Source: three-view drawing plus pictorial views. Frame: mm from the lowest corner of the part. A direction names the side the tool comes from. Give positions to 0.01 mm unless a question says otherwise; leave off trailing zeros. Loops run counter-clockwise (first coordinate to the right, second up) from the corner with the lowest first, then second, coordinate; pieces in that order, holes last. Notation, with made-up numbers: (10, 59) - (33, 59) arc R23 ccw to (33, 95) - close; hole circle Ø5 at (-14, 31.5). An arc over 180 degrees is marked (long way). Answer as a JSON object with one key per item and string values. Group by question number.
(1) Section query A-A (y = 12). Return loops of the section in (x, z), plus the area to 3 significant figures.
(2) Pin query (flat end, axial travel): P1, Ø1.5, axis at y = 7, z = 17, coming from the -X side; P2, Ø4.5, axis at x = 49.5, y = 17, coming from the -Z side; P3, Ø12, axis at x = 30, z = 20, coming from the +Y side. Return the tip coordinate at first contact, or that it passes through.
(3) Access query for the marked faces 1 and 2. Directions: +Z, -Z, +X, -X, +Y, -Y. A direction counts if a zero-diameter tool reaches every point of the face in a straight line with its end or side. Return the directions, or none.
(4) Section query B-B (z = 20). Return loops of the section in (x, y).
(5) Material intervals for L1, parallel to Y at x = 52.5, z = 44.75; L2, parallel to X at y = 19, z = 20; L3, parallel to Z at x = 49, y = 18.5, sorted ascending.
(6) Mould query, pull axis X, two halves, no side actions, for the marked faces 3, 4, 5 and 6. Classes: +X half, -X half, draft (parallel to the pull), parting line (faces both ways), or undercut.
(7) Section query C-C (x = 30). Return loops of the section in (y, z).
(8) Section query D-D (y = 2.75). Return loops of the section in (x, z).
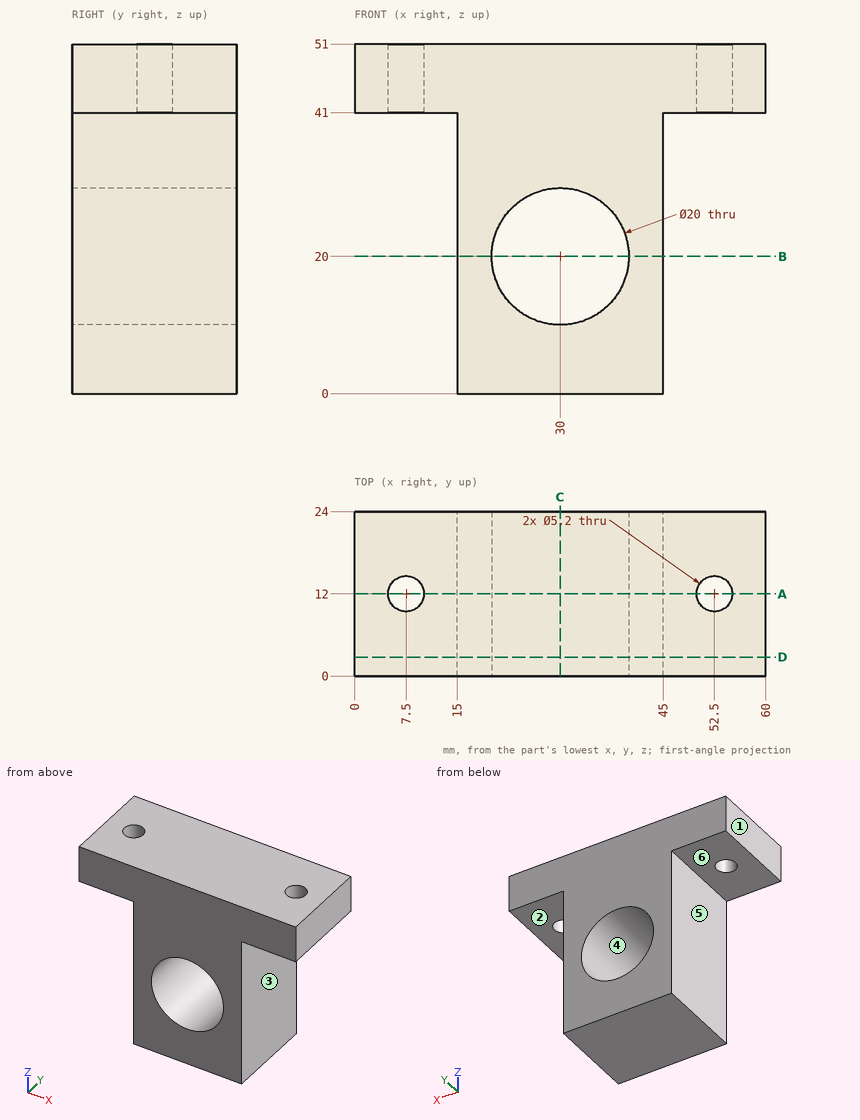
Recorded:
{
 "1": {"outline": "(0, 41) - (4.9, 41) - (4.9, 51) - (0, 51) - close; (10.1, 41) - (15, 41) - (15, 0) - (45, 0) - (45, 41) - (49.9, 41) - (49.9, 51) - (10.1, 51) - close; (55.1, 41) - (60, 41) - (60, 51) - (55.1, 51) - close; hole circle Ø20 at (30, 20)", "area": "1,410 mm^2"},
 "2": {"P1": "stops at x = 15", "P2": "stops at z = 41", "P3": "passes through"},
 "3": {"face 1": "+Z, -Z, -X, +Y, -Y", "face 2": "-Z, +X, +Y, -Y"},
 "4": {"outline": "(15, 0) - (20, 0) - (20, 24) - (15, 24) - close; (40, 0) - (45, 0) - (45, 24) - (40, 24) - close"},
 "5": {"L1": "y = 0 to 9.4, 14.6 to 24", "L2": "x = 15 to 20, 40 to 45", "L3": "z = 41 to 51"},
 "6": {"face 3": "+X half", "face 4": "undercut", "face 5": "-X half", "face 6": "draft"},
 "7": {"outline": "(0, 0) - (24, 0) - (24, 10) - (0, 10) - close; (0, 30) - (24, 30) - (24, 51) - (0, 51) - close"},
 "8": {"outline": "(0, 41) - (15, 41) - (15, 0) - (45, 0) - (45, 41) - (60, 41) - (60, 51) - (0, 51) - close; hole circle Ø20 at (30, 20)"}
}
